from build123d import *

# Parameters (mm, degrees)
EXTRUDE_1_DEPTH = 8
FILLET_1_R      = 1


with BuildPart() as part:
    # Эскиз1 → Бобышка-Вытянуть1 (new body)
    with BuildSketch(Plane.XY):
        with BuildLine():
            Line((-8.5, 21), (18, 21))
            ThreePointArc((18, 21), (20.121320344, 20.121320344), (21, 18))
            Line((21, 18), (21, -8.5))
            Line((21, -8.5), (18.5, -11))
            Line((18.5, -11), (17, -11))
            Line((17, -11), (17, 0))
            ThreePointArc((17, 0), (12.02081528, 12.02081528), (0, 17))
            Line((0, 17), (-11, 17))
            Line((-11, 17), (-11, 18.5))
            Line((-11, 18.5), (-8.5, 21))
        make_face()
    extrude(amount=EXTRUDE_1_DEPTH)

    # Скругление1
    fillet_1_edges = [part.edges().sort_by_distance(p)[0] for p in [
        (21, 4.75, 0),
        (-11, 17.75, 0),
        (-9.75, 19.75, 0),
        (17.75, -11, 8),
        (19.75, -9.75, 8),
        (21, 4.75, 8),
        (20.121320344, 20.121320344, 8),
        (4.75, 21, 8),
        (-9.75, 19.75, 8),
        (-11, 17.75, 8),
        (4.75, 21, 0),
        (20.121320344, 20.121320344, 0),
    ]]
    fillet(fillet_1_edges, radius=FILLET_1_R)


solid = part.part
Can you work these out from the model? Positions are in its coordinate system, mm. A direction names the side the tool comes from. Coordinates: 2 decimals unless noted, no trailing zeros. Order: outer loops, then holes, each group sorted by start corner. A loop starts at its lowest first (then second) coordinate and runs counter-clockwise, first axis right, second up. Notation, with made-up numbers: (37.25, -13.75) - (90.25, -13.75) arc R33 ccw to (90.25, 19.25) - close; hole circle Ø6 at (25.25, 83.25). An arc over 180 degrees is marked (long way). Answer as a JSON object with one key per item and string values. Group by question number.
Q1. Imagine slicing it at D-D (z = 7.5). Please give me the cut outline in (x, y).
Q2. Imagine slicing it at C-C (x = 2). Please give me the cut outline in (y, z), and give its area (3 significant figures).
Q3. Imagine slicing it at A-A (z = 2.5). Please give me the cut outline in (x, y).
Q4. I need wall thicknesses on line 1 (X direction, y = -3, z = 3.25); line 2 (Y direction, x = 10, z = 3.75). Which ranges of each line are inside material? Lowest first, please. Write a range as from..to.
Q5. Imagine slicing it at B-B (y = -5.5). Please give me the cut outline in (x, z).
Q6. On a 3-axis mill with a long thin cutter (end or side, diameter ignored), from which of +Z, -Z, +X, -X, +Y, -Y can I reach the whole of each face in a straight line? I mean faces 1 (the face through (20.715, 4.565, 7.699)), 2 (the face through (17, -6, 4)). Say none if no direction works.
Q7. Will these pins go through, and if not, where does the flat tip stop? P1, Ø2, axis at y = 10.5, z = 4, coming from the -X side; P2, Ø4, axis at x = -7.5, z = 5.5, coming from the -Y side; P3, Ø1.5, axis at y = 14, z = 3.5, coming from the -X side.
Determined:
{
 "1": {"outline": "(-10.87, 17) - (0, 17) arc R17 cw to (17, 0) - (17, -10.87) - (18.44, -10.87) - (20.87, -8.44) - (20.87, 18) arc R2.87 ccw to (18, 20.87) - (-8.44, 20.87) - (-10.87, 18.44) - close"},
 "2": {"outline": "(16.88, 0) - (20, 0) arc R1 ccw to (21, 1) - (21, 7) arc R1 ccw to (20, 8) - (16.88, 8) - close", "area": "32.5 mm2"},
 "3": {"outline": "(-11, 17) - (0, 17) arc R17 cw to (17, 0) - (17, -11) - (18.5, -11) - (21, -8.5) - (21, 18) arc R3 ccw to (18, 21) - (-8.5, 21) - (-11, 18.5) - close"},
 "4": {"line 1": "x = 17..21", "line 2": "y = 13.75..21"},
 "5": {"outline": "(17, 0) - (20, 0) arc R1 ccw to (21, 1) - (21, 7) arc R1 ccw to (20, 8) - (17, 8) - close"},
 "6": {"face 1": "+Z, +X, +Y, -Y", "face 2": "+Z, -Z, -X, -Y"},
 "7": {"P1": "stops at x = 12.52", "P2": "stops at y = 17", "P3": "stops at x = 8.45"}
}
